```python
from build123d import *

# Parameters (mm, degrees)
SKETCH1_R           = 20
BOSS_EXTRUDE1_DEPTH = 2
SKETCH2_R           = 17.2
BOSS_EXTRUDE2_DEPTH = 6.5
CUT_EXTRUDE1_DEPTH  = 30.533878851


with BuildPart() as part:
    # Sketch1 → Boss-Extrude1 (new body)
    with BuildSketch(Plane.XY):
        Circle(SKETCH1_R)
    extrude(amount=BOSS_EXTRUDE1_DEPTH)

    # Sketch2 → Boss-Extrude2 (add)
    with BuildSketch(Plane.XY.offset(2)):
        with Locations(Location((0, 0, 0), (0, 0, 180))):
            Circle(SKETCH2_R)
    extrude(amount=BOSS_EXTRUDE2_DEPTH)

    # Sketch3 → Cut-Extrude1 (cut, through all)
    with BuildSketch(Plane.XY.offset(8.5)):
        Polygon((0, 11.547005384), (-10, 5.773502692), (-10, -5.773502692), (0, -11.547005384), (10, -5.773502692), (10, 5.773502692), align=None)
    extrude(amount=-CUT_EXTRUDE1_DEPTH, mode=Mode.SUBTRACT)


solid = part.part
```
Design review of the part built by this model. Coordinates are the model's own, in mm. A direction names the side the tool comes from. Round coordinates to 2 decimals unless told otherwise and drop trailing zeros. Write each loop counter-clockwise with the first axis right and the second up, starting at its lowest first coordinate (ties: lowest second). Pieces come first, ordered by that corner, then holes. Notation, with made-up numbers: (-23, 58.5) -> (-18, 58.5) arc R13 ccw to (-18, 74.5) -> close; hole circle Ø4 at (17, 34.5). An arc over 180 degrees is marked (long way). Answer in a Markdown table with one row per item.
Q1. Draft analysis for pull direction Z (two halves, no side actions). For faces 3 (the face through (-5, 9, 0)), 4 (the face through (4.93, -8.7, 4.31)), 5 (the face through (-7, -8, 8.5)), state which applies: +Z half, -Z half, draft (parallel to the pull), parting line (faces both ways), or undercut.
The answers:
| item | result |
|---|---|
| face 3 | -Z half |
| face 4 | draft |
| face 5 | +Z half |
Q2. Clearance check with flat-ended pins moving along their axes: pin 1 Ø2 at (x, z) = (-14.5, 2.5) entering from +Y; pin 2 Ø4 at (y, z) = (-14, 5.5) entering from +X; pin 3 Ø1.5 at (x, z) = (-9.5, 2) entering from +Y. State where each tip first meets the part, or that it passes through.
The answers:
| item | result |
|---|---|
| pin 1 | y = 14.63 |
| pin 2 | x = 12.32 |
| pin 3 | y = 17.98 |
Q3. Take a section at A-A, the plane y = 0. State the section outline as (x, z) points.
The answers:
| item | result |
|---|---|
| outline | (-20, 0) -> (-10, 0) -> (-10, 8.5) -> (-17.2, 8.5) -> (-17.2, 2) -> (-20, 2) -> close; (10, 0) -> (20, 0) -> (20, 2) -> (17.2, 2) -> (17.2, 8.5) -> (10, 8.5) -> close |
Q4. To check wall thickness, follow L1, parallel to Y at x = 0, z = 3; L2, parallel to X at y = -3, z = 7.5; L3, parallel to Y at x = -1.5, z = 7.5. State the ranges of each line that lie inside material, in increasing order. Write a range as [from, to].
The answers:
| item | result |
|---|---|
| L1 | [-17.2, -11.55], [11.55, 17.2] |
| L2 | [-16.94, -10], [10, 16.94] |
| L3 | [-17.13, -10.68], [10.68, 17.13] |
Q5. Take a section at C-C, the plane x = 5. State the section outline as (y, z) points.
The answers:
| item | result |
|---|---|
| outline | (-19.36, 0) -> (-8.66, 0) -> (-8.66, 8.5) -> (-16.46, 8.5) -> (-16.46, 2) -> (-19.36, 2) -> close; (8.66, 0) -> (19.36, 0) -> (19.36, 2) -> (16.46, 2) -> (16.46, 8.5) -> (8.66, 8.5) -> close |
Q6. For faces 1 (the face through (9, 15, 2)), 2 (the face through (10, 0, 4)), list the 3-axis set-ups (+Z, -Z, +X, -X, +Y, -Y) from which the entire face can be reached by the end or side of a thin tool; tool diameter is ignored.
The answers:
| item | result |
|---|---|
| face 1 | +Z |
| face 2 | +Z, -Z |
Q7. Take a section at B-B, the plane z = 2.75. State the section outline as (x, y) points.
The answers:
| item | result |
|---|---|
| outline | circle Ø34.4 at (0, 0); hole (-10, -5.77) -> (0, -11.55) -> (10, -5.77) -> (10, 5.77) -> (0, 11.55) -> (-10, 5.77) -> close |
